For this review, take the finished solid that the model builds, in its own axes (mm). A direction names the side the tool comes from. Coordinates: 2 decimals unless noted, no trailing zeros. Order: outer loops, then holes, each group sorted by start corner. A loop starts at its lowest first (then second) coordinate and runs counter-clockwise, first axis right, second up. Notation, with made-up numbers: M 83.5,56 L 115.5,56 A19 ccw 115.5,71 Z; hole C 66.25,-29 d5. An arc over 180 degrees is marked long. Use one line per item in the form item = value. Start each with the question number.
```python
from build123d import *

# Parameters (mm, degrees)
F0_W     = 279.4
F0_H     = 139.7
F1_DEPTH = 19.05
F2_W     = 127
F2_H     = 19.05
F3_DEPTH = 139.7
F4_W     = 139.7
F4_H     = 19.05
F5_DEPTH = 139.7
F6_R     = 3.96875
F7_DEPTH = 139.7
F8_R     = 5.08
F9_DEPTH = 50.8


with BuildPart() as f1:
    # F0 (on Top) → F1 (new body)
    with BuildSketch(Plane.XY):
        with Locations((139.7, 69.85)):
            Rectangle(F0_W, F0_H)
    extrude(amount=F1_DEPTH)

    # F2 (on face) → F3 (join)
    with BuildSketch(Plane.XY.offset(19.05)):
        with Locations((63.5, 130.175)):
            Rectangle(F2_W, F2_H)
    extrude(amount=F3_DEPTH)

    # F4 (on face) → F5 (join)
    with BuildSketch(Plane.XY.offset(19.05)):
        with Locations((69.85, 9.525)):
            Rectangle(F4_W, F4_H)
    extrude(amount=F5_DEPTH)

    # F6 (on face) → F7 (join, through all)
    with BuildSketch(Plane.XZ):
        with Locations((69.85, 88.9)):
            Circle(F6_R)
    extrude(amount=-F7_DEPTH)

    # F8
    f8_edges = [f1.edges().sort_by_distance(p)[0] for p in [
        (139.7, 9.525, 158.75),
        (0, 9.525, 158.75),
        (0, 130.175, 158.75),
        (127, 130.175, 158.75),
        (279.4, 0, 9.525),
        (279.4, 139.7, 9.525),
        (279.4, 69.85, 19.05),
    ]]
    fillet(f8_edges, radius=F8_R)

    # F9 (add): a face of the model
    f9_faces = [f1.faces().sort_by_distance(p)[0] for p in [
        (139.6606680243, 69.85, 0),
    ]]
    extrude(f9_faces, amount=F9_DEPTH)


solid = f1.part
```
1. Consider section D-D, the plane z = 88.9. Write out the cut boundary in (x, y), plus the area to 3 significant figures.
2. Consider section A-A, the plane y = 50. Write out the cut boundary in (x, z).
3. Consider section B-B, the plane z = 38.5. Write out the cut boundary in (x, y), plus the area to 3 significant figures.
4. To check wall thickness, follow line 1 (Y direction, x = 121, z = 89.5); line 2 (X direction, y = 15, z = 116.5); line 3 (Z direction, x = 55.5, y = 107.5). State the ranges of each line that lie inside material, in increasing order.
5. Tool access review of faces 1 (the cylindrical face through (68.99, 69.139, 85.026)), 2 (the flat face through (139.7, 9, 85)), 3 (the flat face through (127, 130, 85)): name each direction out of +Z, -Z, +X, -X, +Y, -Y from which nothing blocks a thin tool from reaching the whole face with its end or side.
6. Consider section C-C, the plane x = 69.85. Write out the cut boundary in (y, z), plus the area to 3 significant figures.
7. The part is to be moulded in two halves that separate along Y. For faces 4 (the flat face through (63, 120.65, 88)), 5 (the flat face through (105, 139.7, 32)), 6 (the flat face through (279.4, 69, -18)), 7 (the flat face through (84, 19.05, 88)), say which applies: pulls with the +Y half, pulls with the -Y half, needs draft (parallel to the pull), parting line crosses it, or undercut.
8. For pin 1 Ø5 at (x, z) = (141.5, 102.5) entering from -Y; pin 2 Ø5 at (y, z) = (24, 46.5) entering from +X; pin 3 Ø21 at (y, z) = (7.5, 72) entering from +X; pin 4 Ø5.5 at (y, z) = (130.5, 103.5) entering from +X, all flat-tipped, find the tip position at first contact; note any pin that passes through.
Answers follow:
q1.outline = M 0,0 L 139.7,0 L 139.7,19.05 L 73.82,19.05 L 73.82,120.65 L 127,120.65 L 127,139.7 L 0,139.7 L 0,120.65 L 65.88,120.65 L 65.88,19.05 L 0,19.05 Z
q1.area = 5,890 mm²
q2.outline = M 0,-50.8 L 279.4,-50.8 L 279.4,13.97 A5.08 ccw 274.32,19.05 L 0,19.05 Z; C 69.85,88.9 d7.94
q3.outline = M 0,0 L 139.7,0 L 139.7,19.05 L 0,19.05 Z; M 0,120.65 L 127,120.65 L 127,139.7 L 0,139.7 Z
q3.area = 5,080 mm²
q4.line_1 = 0 to 19.05, 120.65 to 139.7
q4.line_2 = 0 to 139.7
q4.line_3 = -50.8 to 19.05
q5.face_1 = none
q5.face_2 = +Z, +X, +Y, -Y
q5.face_3 = +Z, +X, +Y
q6.outline = M 0,-50.8 L 139.7,-50.8 L 139.7,158.75 L 120.65,158.75 L 120.65,92.87 L 19.05,92.87 L 19.05,158.75 L 0,158.75 Z; hole M 19.05,19.05 L 120.65,19.05 L 120.65,84.93 L 19.05,84.93 Z
q6.area = 15,900 mm²
q7.face_4 = undercut
q7.face_5 = pulls with the +Y half
q7.face_6 = needs draft
q7.face_7 = undercut
q8.pin_1 = 0
q8.pin_2 = through
q8.pin_3 = 139.7
q8.pin_4 = 127
